Source: CAD feature listing. Evaluate the final solid. Frame: model axes, mm. Coordinates: 2 decimals unless noted, no trailing zeros. Write each loop counter-clockwise with the first axis right and the second up, starting at its lowest first coordinate (ties: lowest second). Pieces come first, ordered by that corner, then holes. Notation, with made-up numbers: M -25.75,74.5 L 19.25,74.5 A19 ccw 19.25,98.5 Z; hole C 27.25,62 d6. An arc over 180 degrees is marked long. Answer as CSV lines item,"result". Start each with the question number.
1. Section C-C on x = -78. Return the cut outline in (y, z).
2. Section A-A on z = -27. Return the cut outline in (x, y).
3. Section B-B on y = 1.4. Return the cut outline in (x, z), plus the area to 3 significant figures.
4. Contact query for flat-ended pins moving along their axis: pin 1 Ø1.5 at (x, y) = (105, 2) entering from -Z; pin 2 Ø1.5 at (y, z) = (1, -4.5) entering from +X; pin 3 Ø1.5 at (x, y) = (-105.5, 2) entering from +Z. Output: stop coordinate, or through.
5. Line query: probe 1 along X at (y, z) = (2.4, -89); probe 2 along Z at (x, y) = (10, 0.2); probe 3 along X at (y, z) = (1.5, -9). Output: solid intervals per line, ascending. Write a range as [from, to].
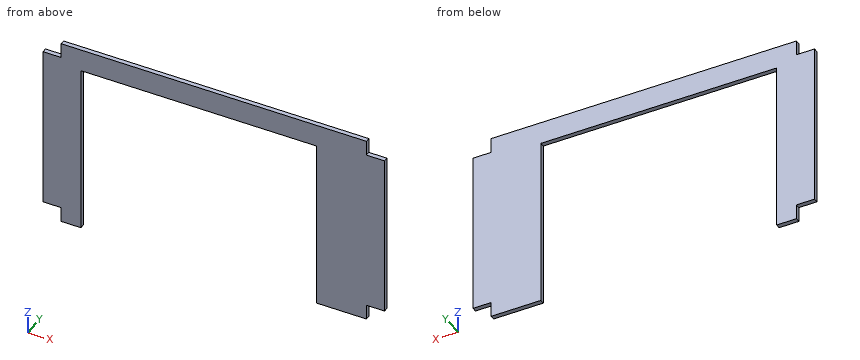
```python
from build123d import *

# Parameters (mm, degrees)
SKETCH1_W           = 225.24
SKETCH1_H           = 129
BOSS_EXTRUDE1_DEPTH = 3
SKETCH2_W           = 12
SKETCH2_H           = 10
SKETCH2_W_2         = 155.5
SKETCH2_H_2         = 114
CUT_EXTRUDE1_DEPTH  = 172.269566473


with BuildPart() as part:
    # Sketch1 → Boss-Extrude1 (new body)
    with BuildSketch(Plane(origin=(0, 0, 0), x_dir=(1, 0, 0), z_dir=(0, 1, 0))):
        with Locations((0, 64.5)):
            Rectangle(SKETCH1_W, SKETCH1_H)
    extrude(amount=BOSS_EXTRUDE1_DEPTH)

    # Sketch2 → Cut-Extrude1 (cut, through all)
    with BuildSketch(Plane(origin=(0, 3, 0), x_dir=(1, 0, 0), z_dir=(0, 1, 0))):
        with Locations((-106.62, 124)):
            Rectangle(SKETCH2_W, SKETCH2_H)
        with Locations((106.62, 124)):
            Rectangle(SKETCH2_W, SKETCH2_H)
        with Locations((106.62, 5)):
            Rectangle(SKETCH2_W, SKETCH2_H)
        with Locations((-106.62, 5)):
            Rectangle(SKETCH2_W, SKETCH2_H)
        with Locations((-9.87, 72)):
            Rectangle(SKETCH2_W_2, SKETCH2_H_2)
    extrude(amount=-CUT_EXTRUDE1_DEPTH, mode=Mode.SUBTRACT)


solid = part.part
```
Values:
1,outline,"M 0,-15 L 3,-15 L 3,0 L 0,0 Z"
2,outline,"M -112.62,0 L -87.62,0 L -87.62,3 L -112.62,3 Z; M 67.88,0 L 112.62,0 L 112.62,3 L 67.88,3 Z"
3,outline,"M -112.62,-119 L -100.62,-119 L -100.62,-129 L -87.62,-129 L -87.62,-15 L 67.88,-15 L 67.88,-129 L 100.62,-129 L 100.62,-119 L 112.62,-119 L 112.62,-10 L 100.62,-10 L 100.62,0 L -100.62,0 L -100.62,-10 L -112.62,-10 Z"
3,area,"10,800 mm²"
4,pin 1,"z = -119"
4,pin 2,"x = 100.62"
4,pin 3,"z = -10"
5,probe 1,"[-112.62, -87.62], [67.88, 112.62]"
5,probe 2,"[-15, 0]"
5,probe 3,"[-100.62, 100.62]"
